Here's how the part is built. I have some questions about the finished solid (model axes, mm). A direction names the side the tool comes from. Give positions to 0.01 mm unless a question says otherwise; leave off trailing zeros. Loops run counter-clockwise (first coordinate to the right, second up) from the corner with the lowest first, then second, coordinate; pieces in that order, holes last.
Q1. Suppose I cut it at C-C (x = 40). List the corners of the cut face in (y, z) for me, and give its area (3 significant figures).
Q2. Suppose I cut it at D-D (z = 53). List the corners of the cut face in (x, y) for me, and give its area (3 significant figures).
Q3. Suppose I cut it at B-B (z = 68). List the corners of the cut face in (x, y) for me.
Q4. I need wall thicknesses on probe 1 along X at (y, z) = (0, 37); probe 2 along X at (y, z) = (3, 27.5); probe 3 along X at (y, z) = (0, 61.5). Which ranges of each line are inside material? Lowest first, please.
Q5. I'm going to push flat-ended pins straight in: P1, Ø23, axis at x = -28.5, z = 23, coming from the -Y side; P2, Ø8, axis at x = -40.5, z = 24.5, coming from the +Y side. Where does each tip first touch, or does it pass through?
Q6. Suppose I cut it at A-A (y = 0). List the corners of the cut face in (x, z) for me.
Q7. Thinking about a two-plate mould opening in X: for faces 4 (the face through (-35.762, -4.03, 37.567)), 5 (the face through (0, -97.658, 57)), 6 (the face through (71.89, -1, 38)), which applies, pulls with the +X half, pulls with the -X half, needs draft (parallel to the pull), parting line crosses it, or undercut?
Q8. For faces 1 (the face through (-1, 72.258, 38)), 2 (the face through (-1, 1, 0)), 3 (the face through (-1, -72.258, 38)), which set-ups out of +Z, -Z, +X, -X, +Y, -Y let a thin tool reach every point of the face, with its end or its side?
```python
from build123d import *

# Parameters (mm, degrees)
F0_W     = 143.7808871269
F0_H     = 144.5161998272
F1_DEPTH = 76.2
F3_DEPTH = 144.5171998272
F5_DEPTH = 25.4
F7_DEPTH = 25.4
F8_R     = 10.5219569488
F9_DEPTH = 101.6


with BuildPart() as f1:
    # F0 (on Top) → F1 (new body)
    with BuildSketch(Plane.XY):
        Rectangle(F0_W, F0_H)
    extrude(amount=F1_DEPTH)

    # F2 (on face) → F3 (cut, through all)
    with BuildSketch(Plane.XZ.offset(72.2580999136)):
        with BuildLine():
            ThreePointArc((-16.4828058332, 76.2), (0, 59.7171941668), (16.4828058332, 76.2))
            Line((16.4828058332, 76.2), (-16.4828058332, 76.2))
        make_face()
    extrude(amount=-F3_DEPTH, mode=Mode.SUBTRACT)

    # F4 (on face) → F5 (join)
    with BuildSketch(Plane.XZ.offset(72.2580999136)):
        with BuildLine():
            Line((-16.4828058332, 76.2), (-26.7050843686, 76.2))
            ThreePointArc((-26.7050843686, 76.2), (0, 49.4949156314), (26.7050843686, 76.2))
            Line((26.7050843686, 76.2), (16.4828058332, 76.2))
            ThreePointArc((16.4828058332, 76.2), (0, 59.7171941668), (-16.4828058332, 76.2))
        make_face()
    extrude(amount=F5_DEPTH)

    # F6 (on face) → F7 (join)
    with BuildSketch(Plane(origin=(0, 72.2580999136, 0), x_dir=(-1, 0, 0), z_dir=(0, 1, 0))):
        with BuildLine():
            ThreePointArc((-26.7050843686, 76.2), (0, 49.4949156314), (26.7050843686, 76.2))
            Line((26.7050843686, 76.2), (16.4828058332, 76.2))
            ThreePointArc((16.4828058332, 76.2), (0, 59.7171941668), (-16.4828058332, 76.2))
            Line((-16.4828058332, 76.2), (-26.7050843686, 76.2))
        make_face()
    extrude(amount=F7_DEPTH)

    # F8 (on Top) → F9 (cut)
    with BuildSketch(Plane.XY):
        with Locations((46.426974237, 0)):
            Circle(F8_R)
        with Locations((-45.4818941653, 0)):
            Circle(F8_R)
    extrude(amount=F9_DEPTH, mode=Mode.SUBTRACT)


solid = f1.part
```
Solutions:
1. outline: (-72.26, 0) - (-8.33, 0) - (-8.33, 76.2) - (-72.26, 76.2) - close; (8.33, 0) - (72.26, 0) - (72.26, 76.2) - (8.33, 76.2) - close
1. area: 9,740 mm2
2. outline: (-71.89, -72.26) - (-13.23, -72.26) - (-13.23, -97.66) - (13.23, -97.66) - (13.23, -72.26) - (71.89, -72.26) - (71.89, 72.26) - (13.23, 72.26) - (13.23, 97.66) - (-13.23, 97.66) - (-13.23, 72.26) - (-71.89, 72.26) - close; hole circle Ø21.04 at (-45.48, 0); hole circle Ø21.04 at (46.43, 0)
2. area: 21,400 mm2
3. outline: (-71.89, -72.26) - (-25.41, -72.26) - (-25.41, -97.66) - (-14.3, -97.66) - (-14.3, 97.66) - (-25.41, 97.66) - (-25.41, 72.26) - (-71.89, 72.26) - close; (14.3, -97.66) - (25.41, -97.66) - (25.41, -72.26) - (71.89, -72.26) - (71.89, 72.26) - (25.41, 72.26) - (25.41, 97.66) - (14.3, 97.66) - close; hole circle Ø21.04 at (-45.48, 0); hole circle Ø21.04 at (46.43, 0)
4. probe 1: x = -71.89 to -56, -34.96 to 35.91, 56.95 to 71.89
4. probe 2: x = -71.89 to -55.57, -35.4 to 36.34, 56.51 to 71.89
4. probe 3: x = -71.89 to -56, -34.96 to -7.46, 7.46 to 35.91, 56.95 to 71.89
5. P1: stops at y = -72.26
5. P2: stops at y = 72.26
6. outline: (-71.89, 0) - (-56, 0) - (-56, 76.2) - (-71.89, 76.2) - close; (-34.96, 0) - (35.91, 0) - (35.91, 76.2) - (16.48, 76.2) arc R16.48 cw to (-16.48, 76.2) - (-34.96, 76.2) - close; (56.95, 0) - (71.89, 0) - (71.89, 76.2) - (56.95, 76.2) - close
7. face 4: undercut
7. face 5: needs draft
7. face 6: pulls with the +X half
8. face 1: -Z, +Y
8. face 2: -Z, +X, -X, +Y, -Y
8. face 3: -Z, -Y
